Geometry check sheet. Reference: drawing and pictorial views, mm from the part's lowest x, y, z. A direction names the side the tool comes from. Coordinates: 2 decimals unless noted, no trailing zeros. Loops run counter-clockwise (first coordinate to the right, second up) from the corner with the lowest first, then second, coordinate; pieces in that order, holes last.
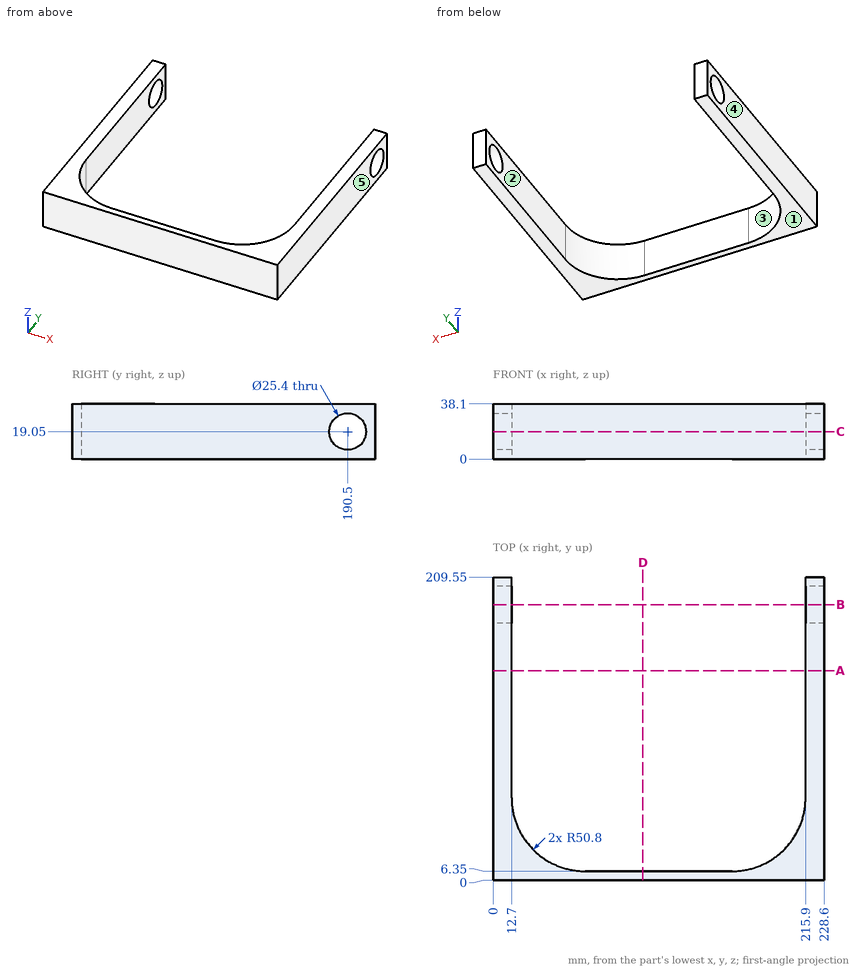
1) Section check C-C on z = 19.05. Record the cut outline in (x, y), and give its area (3 significant figures).
Data:
outline: (0, 0) - (228.6, 0) - (228.6, 177.8) - (215.9, 177.8) - (215.9, 57.15) arc R50.8 cw to (165.1, 6.35) - (63.5, 6.35) arc R50.8 cw to (12.7, 57.15) - (12.7, 177.8) - (0, 177.8) - close; (0, 203.2) - (12.7, 203.2) - (12.7, 209.55) - (0, 209.55) - close; (215.9, 203.2) - (228.6, 203.2) - (228.6, 209.55) - (215.9, 209.55) - close
area: 7,080 mm2
2) Access from +Z, -Z, +X, -X, +Y, -Y to the whole of each face (thin tool, end or side, straight path). Record for the marked faces 1 and 2.
Data:
face 1: -Z, +X, -X, +Y, -Y
face 2: +Z, -Z, +Y
3) Section check B-B on y = 190.5. Record the cut outline in (x, z), and give its area (3 significant figures).
Data:
outline: (0, 0) - (12.7, 0) - (12.7, 6.35) - (0, 6.35) - close; (0, 31.75) - (12.7, 31.75) - (12.7, 38.1) - (0, 38.1) - close; (215.9, 0) - (228.6, 0) - (228.6, 6.35) - (215.9, 6.35) - close; (215.9, 31.75) - (228.6, 31.75) - (228.6, 38.1) - (215.9, 38.1) - close
area: 323 mm2
4) Mould release check, pull along X, two halves, no side actions. Record for the marked faces 3, 4 and 5: +X half, -X half, draft (parallel to the pull), parting line (faces both ways), or undercut.
Data:
face 3: undercut
face 4: -X half
face 5: +X half
5) Section check D-D on x = 103.5. Record the cut outline in (y, z).
Data:
outline: (0, 0) - (6.35, 0) - (6.35, 38.1) - (0, 38.1) - close
6) Material ranges on probe 1 along Y at (x, z) = (221.75, 19.05); probe 2 along X at (y, z) = (157.5, 14); probe 3 along X at (y, z) = (20, 35.5), recorded low to high.
Data:
probe 1: y = 0 to 177.8, 203.2 to 209.55
probe 2: x = 0 to 12.7, 215.9 to 228.6
probe 3: x = 0 to 28.85, 199.75 to 228.6
7) Section check A-A on y = 145. Record the cut outline in (x, z).
Data:
outline: (0, 0) - (12.7, 0) - (12.7, 38.1) - (0, 38.1) - close; (215.9, 0) - (228.6, 0) - (228.6, 38.1) - (215.9, 38.1) - close
8) Depth check by flat-ended pin: pin 1 (5 mm diameter, centred on x = 152, z = 24, fed in from +Y); pin 2 (12 mm diameter, centred on x = 181.5, z = 30.5, fed in from +Y); pin 3 (10 mm diameter, centred on y = 185, z = 12, fed in from +X). Enter the tip coordinate at first touch or a pass-through.
Data:
pin 1: stops at y = 6.35
pin 2: stops at y = 11.56
pin 3: stops at x = 228.6
